Answer from the drawing. Dimensions are ordinates in mm from the lowest x, y and z of the part. A direction names the side the tool comes from. Coordinates: 2 decimals unless noted, no trailing zeros. Write each loop counter-clockwise with the first axis right and the second up, starting at its lowest first coordinate (ties: lowest second). Pieces come first, ordered by that corner, then holes. Notation, with made-up numbers: (70, -38.5) -> (122, -38.5) arc R17 cw to (122, -21.5) -> close; hole circle Ø9 at (11, -37). An arc over 180 degrees is marked (long way). One line per item, written item: value. Start each with the question number.
1. Given P1, Ø1.3, axis at x = 6, y = 21.5, coming from the +Z side; P2, Ø2, axis at x = 4, y = 22, coming from the -Z side; P3, Ø2.5, axis at x = 7.5, z = 29.5, coming from the +Y side; P4, Ø3, axis at x = 8.5, z = 8.5, coming from the -Y side, each flat-ended and moving along its own axis, determine where each tip first touches the part or whether it passes through.
2. Find section C-C, the plane x = 2.5. Write down the section's boundary in (y, z).
3. Find section B-B, the plane z = 10.75. Write down the section's boundary in (x, y).
4. Find section D-D, the plane y = 2. Write down the section's boundary in (x, z), and give its area (3 significant figures).
5. Consider line 1 along Z through (x, y) = (6.1, 18.2); line 2 along Y through (x, z) = (5, 22); line 3 along X through (y, z) = (18, 30). Determine where each line is inside the solid, lowest interval first.
6. For the marked faces 1, 2, 3 and 4, determine the directions among +Z, -Z, +X, -X, +Y, -Y from which every point of the face is accessible in a straight line to the end or side of a thin tool.
7. Find section A-A, the plane z = 2. Write down the section's boundary in (x, y), and give its area (3 significant figures).
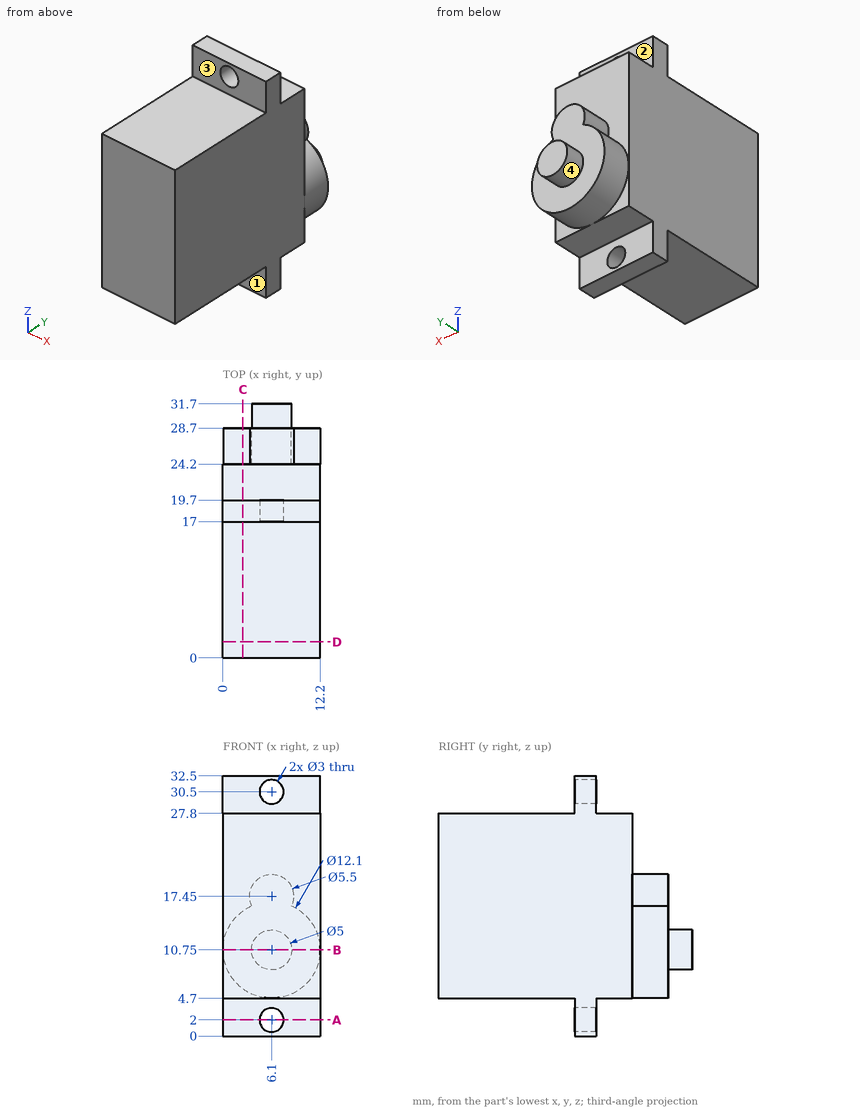
Answer block:
1. P1: stops at z = 27.8
1. P2: stops at z = 4.7
1. P3: stops at y = 19.7
1. P4: stops at y = 0
2. outline: (0, 4.7) -> (17, 4.7) -> (17, 0) -> (19.7, 0) -> (19.7, 4.7) -> (24.2, 4.7) -> (24.2, 5.89) -> (28.7, 5.89) -> (28.7, 15.61) -> (24.2, 15.61) -> (24.2, 27.8) -> (19.7, 27.8) -> (19.7, 32.5) -> (17, 32.5) -> (17, 27.8) -> (0, 27.8) -> close
3. outline: (0, 0) -> (12.2, 0) -> (12.2, 24.2) -> (12.15, 24.2) -> (12.15, 28.7) -> (8.6, 28.7) -> (8.6, 31.7) -> (3.6, 31.7) -> (3.6, 28.7) -> (0.05, 28.7) -> (0.05, 24.2) -> (0, 24.2) -> close
4. outline: (0, 4.7) -> (12.2, 4.7) -> (12.2, 27.8) -> (0, 27.8) -> close
4. area: 282 mm2
5. line 1: z = 0 to 0.5, 3.5 to 29, 32 to 32.5
5. line 2: y = 0 to 24.2
5. line 3: x = 0 to 4.69, 7.51 to 12.2
6. face 1: -Z, +X, -X, -Y
6. face 2: +Z, +X, -X, +Y
6. face 3: +Z, +X, -X, -Y
6. face 4: +Y
7. outline: (0, 17) -> (4.6, 17) -> (4.6, 19.7) -> (0, 19.7) -> close; (7.6, 17) -> (12.2, 17) -> (12.2, 19.7) -> (7.6, 19.7) -> close
7. area: 24.8 mm2
